from build123d import *

# Parameters (mm, degrees)
SKETCH_1_R               = 2.25
EXTRUDE_1_DEPTH          = 104
CHAMFER_1_SIZE           = 1
CUT_EXTRUDE_1_DEPTH      = 105.048666498
CUT_EXTRUDE_1_DEPTH_BACK = 105.048666498
SKETCH_2_R               = 1


with BuildPart() as part:
    # 草圖1 → 填料-伸長1 (new body)
    with BuildSketch(Plane.XY):
        with Locations(Location((0, 0, 0), (0, 0, 180))):
            Circle(SKETCH_1_R)
    extrude(amount=EXTRUDE_1_DEPTH)

    # 導角1
    chamfer_1_edges = [part.edges().sort_by_distance(p)[0] for p in [
        (2.25, 0, 0),
        (2.25, 0, 104),
    ]]
    chamfer(chamfer_1_edges, length=CHAMFER_1_SIZE)

    # 草圖2 → 除料-伸長1 (cut, two sides: drawn at the far end of the back side and taken through both)
    with BuildSketch(Plane(origin=(0, 0, 0), x_dir=(1, 0, 0), z_dir=(0, 1, 0)).offset(-CUT_EXTRUDE_1_DEPTH_BACK)):
        with Locations(Location((0, -3, 0), (0, 0, 270))):
            Circle(SKETCH_2_R)
        with Locations(Location((0, -101, 0), (0, 0, 270))):
            Circle(SKETCH_2_R)
    extrude(amount=CUT_EXTRUDE_1_DEPTH + CUT_EXTRUDE_1_DEPTH_BACK, mode=Mode.SUBTRACT)


solid = part.part
Build history of the part. All positions in model axes, mm. Coordinates: 2 decimals unless noted, no trailing zeros. Order: outer loops, then holes, each group sorted by start corner. A loop starts at its lowest first (then second) coordinate and runs counter-clockwise, first axis right, second up. Notation, with made-up numbers: (82.5, 57.25) - (138.5, 57.25) arc R25 ccw to (138.5, 90.25) - close; hole circle Ø9 at (-34.75, -35.75). An arc over 180 degrees is marked (long way). Write each question's results on one line, items separated by ' | '. Start each with the question number.
Item 1: Band-saw the part on B-B on x = 0. Write the cut outline in (y, z).
Item 2: Mould opens along Z. For faces 1 (the face through (0, 0, 0)), 2 (the face through (0, 0, 4)), 3 (the face through (0, 0, 104)) say: released by +Z, released by -Z, zero draft, split by the parting line, or undercut.
Item 3: Band-saw the part on C-C on z = 78. Write the cut outline in (x, y).
Item 4: Band-saw the part on D-D on z = 101. Write the cut outline in (x, y), and give its area (3 significant figures).
Item 5: Flat gauge pins, fed straight in: pin 1 (1.2 mm diameter, centred on x = 0, z = 101, fed in from -Y); pin 2 (1.5 mm diameter, centred on y = 0.5, z = 64.5, fed in from +X). Where does each tip first touch, or does it go through?
Item 6: Band-saw the part on A-A on y = 0. Write the cut outline in (x, z).
Item 7: Wall check: probe 1 along Z at (x, y) = (0, -0.55); probe 2 along Z at (x, y) = (-0.35, -0.6); probe 3 along Y at (x, z) = (0.15, 12) (3 decimals). Give the ranges that are in metal, low to high. Write a range as [from, to].
Numbers:
1) outline: (-2.25, 1) - (-1.25, 0) - (1.25, 0) - (2.25, 1) - (2.25, 2) - (-2.25, 2) - close; (-2.25, 4) - (2.25, 4) - (2.25, 100) - (-2.25, 100) - close; (-2.25, 102) - (2.25, 102) - (2.25, 103) - (1.25, 104) - (-1.25, 104) - (-2.25, 103) - close
2) face 1: released by -Z | face 2: undercut | face 3: released by +Z
3) outline: circle Ø4.5 at (0, 0)
4) outline: (-1, -2.02) - (-1, 2.02) arc R2.25 ccw to start; (1, -2.02) arc R2.25 ccw to (1, 2.02) - close | area: 7.21 mm^2
5) pin 1: through | pin 2: x = 2.25
6) outline: (-2.25, 1) - (-1.25, 0) - (1.25, 0) - (2.25, 1) - (2.25, 103) - (1.25, 104) - (-1.25, 104) - (-2.25, 103) - close; hole circle Ø2 at (0, 3); hole circle Ø2 at (0, 101)
7) probe 1: [0, 2], [4, 100], [102, 104] | probe 2: [0, 2.06], [3.94, 100.06], [101.94, 104] | probe 3: [-2.245, 2.245]
